Design review of the part built by this model. Coordinates are the model's own, in mm. Coordinates: 2 decimals unless noted, no trailing zeros. Loops run counter-clockwise (first coordinate to the right, second up) from the corner with the lowest first, then second, coordinate; pieces in that order, holes last. Notation, with made-up numbers: (-21, 34.25) -> (29, 34.25) arc R24 ccw to (29, 67.25) -> close; hole circle Ø10 at (0, 9). An arc over 180 degrees is marked (long way). Answer in a Markdown table with one row per item.
```python
from build123d import *

# Parameters (mm, degrees)
F0_W     = 74
F0_H     = 74
F1_DEPTH = 59
F2_T     = -1
F3_W     = 76
F3_H     = 76
F3_W_2   = 74
F3_H_2   = 74
F4_DEPTH = 60
F5_W     = 74
F5_H     = 1
F6_DEPTH = 74


with BuildPart() as f1:
    # F0 (on Top) → F1 (new body)
    with BuildSketch(Plane.XY):
        Rectangle(F0_W, F0_H)
    extrude(amount=F1_DEPTH)

    # F2
    f2_openings = [f1.faces().sort_by_distance(p)[0] for p in [
        (0, 0, 59),
    ]]
    offset(amount=F2_T, openings=f2_openings)

    # F3 (on Top) → F4 (join)
    with BuildSketch(Plane.XY):
        Rectangle(F3_W, F3_H)
        Rectangle(F3_W_2, F3_H_2, mode=Mode.SUBTRACT)
    extrude(amount=F4_DEPTH)

    # F5 (on face) → F6 (join, through all)
    with BuildSketch(Plane.YZ.offset(-37)):
        with Locations((0, 59.5)):
            Rectangle(F5_W, F5_H)
    extrude(amount=F6_DEPTH)


solid = f1.part
```
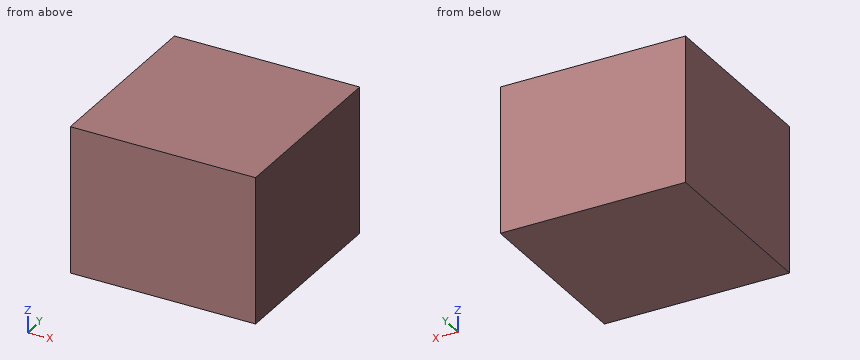
(1) To check wall thickness, follow probe 1 along Y at (x, z) = (18.5, 24.5); probe 2 along Z at (x, y) = (6.5, -14). State the ranges of each line that lie inside material, in increasing order.
Evaluation:
| item | result |
|---|---|
| probe 1 | y = -38 to -36, 36 to 38 |
| probe 2 | z = 0 to 1, 59 to 60 |
(2) Take a section at A-A on y = 22.5. Give the boundary of the cut face in (x, z), and give its area (3 significant figures).
Evaluation:
| item | result |
|---|---|
| outline | (-38, 0) -> (38, 0) -> (38, 60) -> (-38, 60) -> close; hole (-36, 1) -> (36, 1) -> (36, 59) -> (-36, 59) -> close |
| area | 384 mm² |
